For this review, use the dimensioned drawing (mm, ordinates from the lowest corner) and the shaded views. A direction names the side the tool comes from. Give positions to 0.01 mm unless a question says otherwise; leave off trailing zeros. Order: outer loops, then holes, each group sorted by start corner. A loop starts at its lowest first (then second) coordinate and runs counter-clockwise, first axis right, second up. Notation, with made-up numbers: M -20,-38 L -6,-38 A17 ccw -6,-30 Z; hole C 39.25,79.25 d1. An arc over 180 degrees is marked long. One line per question, with ' | ' between items. Start each with the question number.
1. We need section D-D on x = 29. Write out the cut boundary in (y, z), then the cut area to 3 significant figures.
2. Wall thickness on L1, parallel to Z at x = 18.5, y = 34; L2, parallel to Y at x = 23.5, z = 137; L3, parallel to Y at x = 4.5, z = 105.5: over which ranges is each line inside the solid? List them lowest first.
3. We need section C-C on z = 11.5. Write out the cut boundary in (x, y), then the cut area to 3 significant figures.
4. We need section B-B on y = 44. Write out the cut boundary in (x, z), then the cut area to 3 significant figures.
5. We need section A-A on x = 41.5. Write out the cut boundary in (y, z), then the cut area to 4 significant figures.
6. For the marked faces 1, 2, 3, 4 and 5, list the 3-axis set-ups (+Z, -Z, +X, -X, +Y, -Y) from which the entire face can be reached by the end or side of a thin tool; tool diameter is ignored.
7. Insertion check: P1, Ø20, axis at y = 25.5, z = 9, coming from the -X side; P2, Ø7.5, axis at y = 79, z = 144.5, coming from the +X side; P3, Ø8, axis at y = 16, z = 43, coming from the -X side; P4, Ø3.5, axis at y = 81.5, z = 140, coming from the -X side. Each pin has a flat end and moves straight along its axis. Give the tip position at first contact, or say it passes through.
8. The part is to be moulded in two halves that separate along Y. For the marked faces 6, 7 and 8, say which applies: +Y half, -Y half, draft (parallel to the pull), parting line (faces both ways), or undercut.
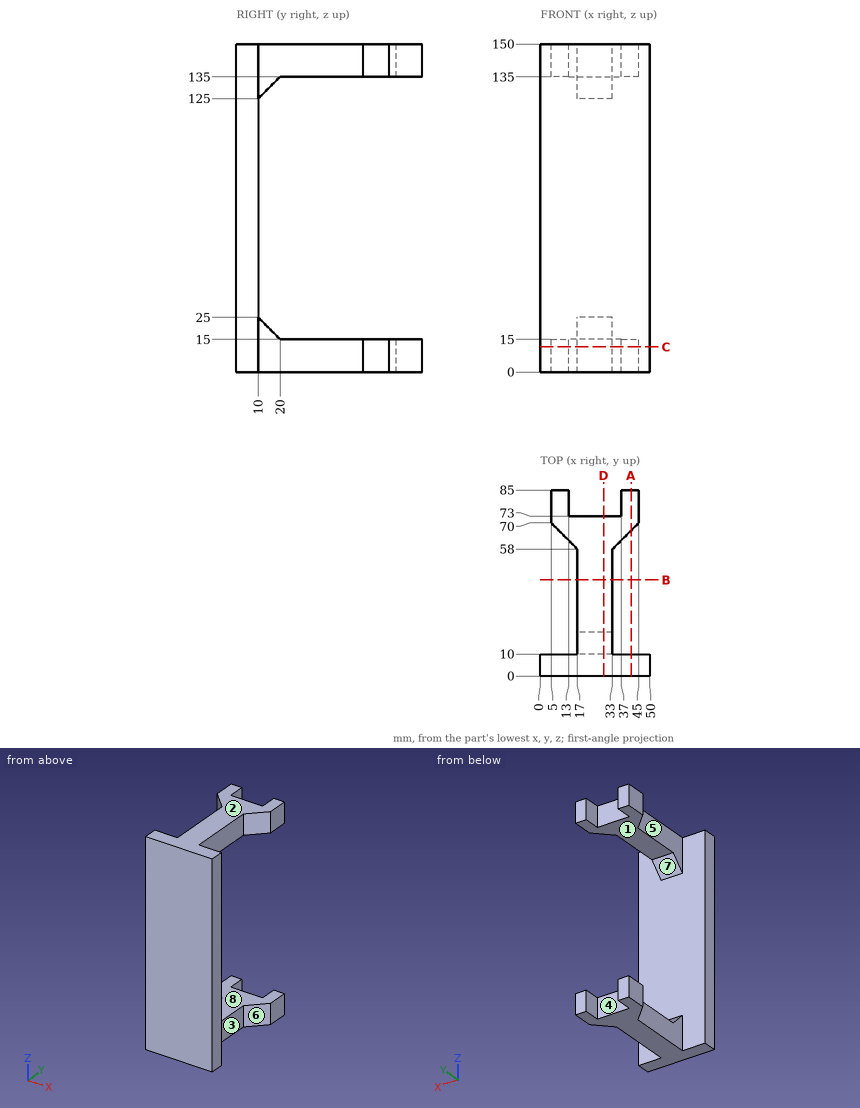
Entries:
1) outline: M 0,0 L 73,0 L 73,15 L 20,15 L 10,25 L 10,125 L 20,135 L 73,135 L 73,150 L 0,150 Z | area: 3,490 mm^2
2) L1: z = 0 to 15, 135 to 150 | L2: y = 0 to 73 | L3: y = 0 to 10
3) outline: M 0,0 L 50,0 L 50,10 L 33,10 L 33,58 L 45,70 L 45,85 L 37,85 L 37,73 L 13,73 L 13,85 L 5,85 L 5,70 L 17,58 L 17,10 L 0,10 Z | area: 1,920 mm^2
4) outline: M 17,0 L 33,0 L 33,15 L 17,15 Z; M 17,135 L 33,135 L 33,150 L 17,150 Z | area: 480 mm^2
5) outline: M 0,0 L 10,0 L 10,150 L 0,150 Z; M 66.5,0 L 85,0 L 85,15 L 66.5,15 Z; M 66.5,135 L 85,135 L 85,150 L 66.5,150 Z | area: 2,055 mm^2
6) face 1: +X, -X, +Y | face 2: +Z, +X, -X, +Y, -Y | face 3: +Z, -Z, +X | face 4: +Z, -Z, +Y | face 5: +Z, -Z, -X
7) P1: stops at x = 17 | P2: stops at x = 45 | P3: passes through | P4: stops at x = 5
8) face 6: undercut | face 7: +Y half | face 8: draft
